from build123d import *

# Parameters (mm, degrees)
F1_DEPTH = 10
F2_R     = 6
F3_DEPTH = 28
F4_SIZE  = 1


with BuildPart() as f1:
    # F0 (on Front) → F1 (new body)
    with BuildSketch(Plane.XZ):
        Polygon((5.731821, -10.023949), (11.546905, -0.048072), (5.815084, 9.975877), (-5.731821, 10.023949), (-11.546905, 0.048072), (-5.815084, -9.975877), align=None)
    extrude(amount=F1_DEPTH)

    # F2 (on face) → F3 (join)
    with BuildSketch(Plane.XZ.offset(10)):
        Circle(F2_R)
    extrude(amount=F3_DEPTH)

    # F4
    f4_edges = [f1.edges().sort_by_distance(p)[0] for p in [
        (-8.639363, 0, 5.036011),
        (0.041632, 0, 9.999913),
        (8.680995, 0, 4.963902),
        (8.639363, 0, -5.036011),
        (-0.041632, 0, -9.999913),
        (-8.680995, 0, -4.963902),
        (-6, -38, 0),
    ]]
    chamfer(f4_edges, length=F4_SIZE)


solid = f1.part
Design review of the part built by this model. Coordinates are the model's own, in mm. A direction names the side the tool comes from. Give positions to 0.01 mm unless a question says otherwise; leave off trailing zeros. Order: outer loops, then holes, each group sorted by start corner. A loop starts at its lowest first (then second) coordinate and runs counter-clockwise, first axis right, second up.
1. To check wall thickness, follow L1, parallel to Y at x = 6.75, z = 4.25; L2, parallel to Z at x = 4.75, y = -3.5; L3, parallel to Z at x = -1, y = -26. State the ranges of each line that lie inside material, in increasing order.
Solution:
L1: y = -10 to 0
L2: z = -10.02 to 9.98
L3: z = -5.92 to 5.92
2. For pin 1 Ø1 at (y, z) = (-10, 6) entering from +X; pin 2 Ø5 at (x, y) = (-3, -32) entering from +Z; pin 3 Ø4 at (x, y) = (7, -29) entering from +Z; pin 4 Ø5 at (y, z) = (-9, -1.5) entering from +X, all flat-tipped, find the tip position at first contact; note any pin that passes through.
Solution:
pin 1: stops at x = 8.37
pin 2: stops at z = 5.98
pin 3: stops at z = 3.32
pin 4: stops at x = 11.55
3. Tool access review of faces 1 (the flat face through (5, -10, 5)), 2 (the flat face through (8.28, -0.49, 4.64)): name each direction out of +Z, -Z, +X, -X, +Y, -Y from which nothing blocks a thin tool from reaching the whole face with its end or side.
Solution:
face 1: -Y
face 2: +Z, +X, +Y
4. Add section C-C, the plane x = -10. State the section outline as (y, z) points, then the cut area to 3 significant figures.
Solution:
outline: (-10, -2.66) - (-1, -2.66) - (0, -0.64) - (0, 0.72) - (-1, 2.7) - (-10, 2.7) - close
area: 51.6 mm2
5. Add section A-A, the plane y = -6.5. State the section outline as (x, z) points, then the cut area to 3 significant figures.
Solution:
outline: (-11.55, 0.05) - (-5.82, -9.98) - (5.73, -10.02) - (11.55, -0.05) - (5.82, 9.98) - (-5.73, 10.02) - close
area: 346 mm2
6. Add section B-B, the plane x = 0. State the section outline as (y, z) points, then the cut area to 3 significant figures.
Solution:
outline: (-38, -5) - (-37, -6) - (-10, -6) - (-10, -10) - (-1, -10) - (0, -9) - (0, 9) - (-1, 10) - (-10, 10) - (-10, 6) - (-37, 6) - (-38, 5) - close
area: 534 mm2
7. Add section D-D, the plane y = -26. State the section outline as (x, z) points.
Solution:
outline: circle Ø12 at (0, 0)
